Here's how the part is built. I have some questions about the finished solid (model axes, mm). Round coordinates to 2 decimals unless told otherwise and drop trailing zeros. Order: outer loops, then holes, each group sorted by start corner. A loop starts at its lowest first (then second) coordinate and runs counter-clockwise, first axis right, second up. Notation, with made-up numbers: (-9.75, 57.5) -> (43.25, 57.5) arc R22 ccw to (43.25, 82.5) -> close; hole circle Ø4 at (0, 41). An arc over 180 degrees is marked (long way). One line per item, written item: value.
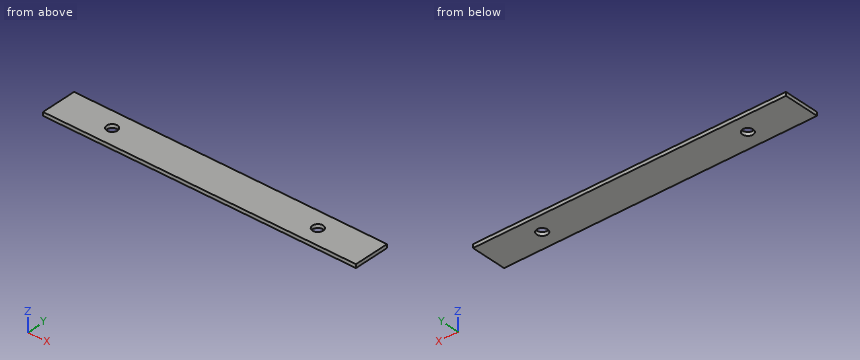
```python
from build123d import *

# Parameters (mm, degrees)
SKETCH_1_W          = 350
SKETCH_1_H          = 40
EXTRUDE_1_DEPTH     = 4
SKETCH_2_R          = 6
CUT_EXTRUDE_1_DEPTH = 353.301007662
SKETCH_3_R          = 6
CUT_EXTRUDE_2_DEPTH = 353.301007662


with BuildPart() as part:
    # Эскиз1 → Бобышка-Вытянуть1 (new body)
    with BuildSketch(Plane.XY):
        with Locations((175, 20)):
            Rectangle(SKETCH_1_W, SKETCH_1_H)
    extrude(amount=EXTRUDE_1_DEPTH)

    # Эскиз2 → Вырез-Вытянуть1 (cut, through all)
    with BuildSketch(Plane.XY.offset(4)):
        with Locations((60, 20)):
            Circle(SKETCH_2_R)
    extrude(amount=-CUT_EXTRUDE_1_DEPTH, mode=Mode.SUBTRACT)

    # Эскиз3 → Вырез-Вытянуть2 (cut, through all)
    with BuildSketch(Plane.XY.offset(4)):
        with Locations((290, 20)):
            Circle(SKETCH_3_R)
    extrude(amount=-CUT_EXTRUDE_2_DEPTH, mode=Mode.SUBTRACT)


solid = part.part
```
Q1. I want a section at B-B on x = 290. Write out the boundary of the cut face in (y, z).
Answers:
outline: (0, 0) -> (14, 0) -> (14, 4) -> (0, 4) -> close; (26, 0) -> (40, 0) -> (40, 4) -> (26, 4) -> close
Q2. I need wall thicknesses on line 1 along Y through (x, z) = (290, 2.55); line 2 along X through (y, z) = (22, 0.5); line 3 along X through (y, z) = (19, 2.25). Which ranges of each line are inside material? Lowest first, please.
Answers:
line 1: 0 to 14, 26 to 40
line 2: 0 to 54.34, 65.66 to 284.34, 295.66 to 350
line 3: 0 to 54.08, 65.92 to 284.08, 295.92 to 350
Q3. For P1, Ø9.5, axis at x = 60, y = 20, coming from the +Z side, with a flat end and sliding along its axis, tell me the tip position at first contact or that it passes through.
Answers:
P1: through
Q4. I want a section at A-A on y = 20. Write out the boundary of the cut face in (x, z).
Answers:
outline: (0, 0) -> (54, 0) -> (54, 4) -> (0, 4) -> close; (66, 0) -> (284, 0) -> (284, 4) -> (66, 4) -> close; (296, 0) -> (350, 0) -> (350, 4) -> (296, 4) -> close
Q5. I want a section at D-D on x = 59. Write out the boundary of the cut face in (y, z), then the cut area to 3 significant figures.
Answers:
outline: (0, 0) -> (14.08, 0) -> (14.08, 4) -> (0, 4) -> close; (25.92, 0) -> (40, 0) -> (40, 4) -> (25.92, 4) -> close
area: 113 mm2
Q6. I want a section at C-C on z = 0.7. Write out the boundary of the cut face in (x, y), then the cut area to 3 significant figures.
Answers:
outline: (0, 0) -> (350, 0) -> (350, 40) -> (0, 40) -> close; hole circle Ø12 at (60, 20); hole circle Ø12 at (290, 20)
area: 13,800 mm2
